from build123d import *

# Parameters (mm, degrees)
F1_DEPTH = 57
F3_D     = 14
F3_DEPTH = 16
F3_TIP   = 4.2060243332


with BuildPart() as f1:
    # F0 (on Front) → F1 (new body)
    with BuildSketch(Plane.XZ):
        Polygon((121, 54), (0, 54), (0, 0), (22, 0), (121, 32), align=None)
    extrude(amount=F1_DEPTH)

    # F3
    with Locations(Plane.XY.offset(54)):
        with Locations((35.2015122771, -16), (68.2015122771, -45)):
            Hole(F3_D / 2, depth=F3_DEPTH)
            with Locations((0, 0, -(F3_DEPTH + F3_TIP / 2))):  # 118° drill point
                Cone(0, F3_D / 2, F3_TIP, mode=Mode.SUBTRACT)


solid = f1.part
Design review of the part built by this model. Coordinates are the model's own, in mm. A direction names the side the tool comes from. Coordinates: 2 decimals unless noted, no trailing zeros. Loops run counter-clockwise (first coordinate to the right, second up) from the corner with the lowest first, then second, coordinate; pieces in that order, holes last. Notation, with made-up numbers: (77.25, -1.5) - (85.25, -1.5) arc R19 cw to (85.25, 27.5) - close; hole circle Ø6 at (-32.5, -1.75). An arc over 180 degrees is marked (long way). Use CSV: the item, a comma, the result in double quotes. Start each with the question number.
1. Mouldability with a two-part tool opening along Y and no side actions: class faces 1 (the flat face through (46, -57, 33)), 2 (the conical face through (67.31, -44.18, 34.52)), 3 (the cylindrical face through (61.525, -42.897, 45.888)), 4 (the flat face through (0, -28, 27)) as released by +Y, released by -Y, zero draft, split by the parting line, or undercut.
2. To check wall thickness, follow probe 1 along X at (y, z) = (-16, 50.5); probe 2 along X at (y, z) = (-45, 47); probe 3 along Z at (x, y) = (98.5, -6.5). State the ranges of each line that lie inside material, in increasing order.
3. Add section C-C on x = 53. Give the boundary of the cut face in (y, z).
4. Add section B-B on z = 30. Give the boundary of the cut face in (x, y).
5. Clearance check with a flat-ended pin moving along its axis: pin 1 (8.5 mm diameter, centred on x = 35.2, y = -16, fed in from -Z). State where the tip first meets the part, or that it passes through.
6. For faces 5 (the cylindrical face through (28.735, -18.681, 45.888)), 6 (the flat face through (46, 0, 33)), list the 3-axis set-ups (+Z, -Z, +X, -X, +Y, -Y) from which the entire face can be reached by the end or side of a thin tool; tool diameter is ignored.
7. Add section A-A on z = 50. Give the boundary of the cut face in (x, y), plus the area to 3 significant figures.
Resolved:
1,face 1,"released by -Y"
1,face 2,"undercut"
1,face 3,"undercut"
1,face 4,"zero draft"
2,probe 1,"0 to 28.2, 42.2 to 121"
2,probe 2,"0 to 61.2, 75.2 to 121"
2,probe 3,"24.73 to 54"
3,outline,"(-57, 10.02) - (0, 10.02) - (0, 54) - (-57, 54) - close"
4,outline,"(0, -57) - (114.81, -57) - (114.81, 0) - (0, 0) - close"
5,pin 1,"z = 2.89"
6,face 5,"+Z"
6,face 6,"+Z, -Z, +X, -X, +Y"
7,outline,"(0, -57) - (121, -57) - (121, 0) - (0, 0) - close; hole circle Ø14 at (35.2, -16); hole circle Ø14 at (68.2, -45)"
7,area,"6,590 mm2"
